Part model, mm, in its own coordinate system. Face numbers are marked on the shaded views. A direction names the side the tool comes from. Round coordinates to 2 decimals unless told otherwise and drop trailing zeros. Order: outer loops, then holes, each group sorted by start corner. A loop starts at its lowest first (then second) coordinate and runs counter-clockwise, first axis right, second up. Notation, with made-up numbers: M 50,1 L 63,1 A22 ccw 63,21 Z; hole C 58.5,-32.5 d7. An arc over 180 degrees is marked long. Write each question's results on one line, items separated by ' | '. Start each with the question number.
1. Band-saw the part on A-A, the plane y = 25. Give the number of separate pieces and of enclosed holes in the cut face, then the cut area to 3 significant figures.
2. Band-saw the part on B-B, the plane x = 107. List the corners of the cut face in (y, z).
3. Band-saw the part on C-C, the plane z = -24. List the corners of the cut face in (x, y).
4. Which spindle directions (+Z, -Z, +X, -X, +Y, -Y) get a long thin tool onto all of the face, cutting with end or side? Do the marked faces 4 and 5. Say none if no direction does.
5. Two-plate mould, pull along Z, no slides. Class the marked faces 1, 2 and 3: +Z half, -Z half, draft (parallel to the pull), parting line (faces both ways), or undercut.
6. Probe L1, parallel to X at y = 13, z = -10.5; L2, parallel to Z at x = 129.5, y = 12; L3, parallel to Z at x = 43, y = 36.5. List the from-to ranges inside material, lowest first. Write a range as [from, to].
7. Drop flat-ended pins along their axis: pin 1 Ø20 at (y, z) = (16, -57.5) entering from -X; pin 2 Ø2.5 at (x, z) = (10.5, -10.5) entering from +Y; pin 3 Ø3 at (x, z) = (-3.5, -42.5) entering from +Y; pin 4 Ø1.8 at (x, z) = (145, -45) entering from -Y. Give the stop position or say it passes through.
```python
from build123d import *

# Parameters (mm, degrees)
SKETCH1_W           = 140
SKETCH1_H           = 90
BOSS_EXTRUDE1_DEPTH = 40
SKETCH2_W           = 135
SKETCH2_H           = 85
CUT_EXTRUDE1_DEPTH  = 37.5
SKETCH3_R           = 3.5
BOSS_EXTRUDE2_DEPTH = 37.5
SKETCH4_R           = 1.5
CUT_EXTRUDE2_DEPTH  = 37.5
BOSS_EXTRUDE3_DEPTH = 3
SKETCH7_R           = 1.5
CUT_EXTRUDE3_DEPTH  = 180.443584449


with BuildPart() as part:
    # Sketch1 → Boss-Extrude1 (new body)
    with BuildSketch(Plane(origin=(0, 0, 0), x_dir=(1, 0, 0), z_dir=(0, 1, 0))):
        with Locations((70, 45)):
            Rectangle(SKETCH1_W, SKETCH1_H)
    extrude(amount=BOSS_EXTRUDE1_DEPTH)

    # Sketch2 → Cut-Extrude1 (cut)
    with BuildSketch(Plane(origin=(0, 40, 0), x_dir=(1, 0, 0), z_dir=(0, 1, 0))):
        with Locations((70, 45)):
            Rectangle(SKETCH2_W, SKETCH2_H)
    extrude(amount=-CUT_EXTRUDE1_DEPTH, mode=Mode.SUBTRACT)

    # Sketch3 → Boss-Extrude2 (add)
    with BuildSketch(Plane(origin=(0, 2.5, 0), x_dir=(1, 0, 0), z_dir=(0, 1, 0))):
        with Locations(Location((10.5, 79.5, 0), (0, 0, 270))):
            Circle(SKETCH3_R)
        with Locations(Location((10.5, 10.5, 0), (0, 0, 270))):
            Circle(SKETCH3_R)
        with Locations(Location((129.5, 10.5, 0), (0, 0, 270))):
            Circle(SKETCH3_R)
        with Locations(Location((129.5, 79.5, 0), (0, 0, 270))):
            Circle(SKETCH3_R)
    extrude(amount=BOSS_EXTRUDE2_DEPTH)

    # Sketch4 → Cut-Extrude2 (cut)
    with BuildSketch(Plane(origin=(0, 40, 0), x_dir=(1, 0, 0), z_dir=(0, 1, 0))):
        with Locations(Location((10.5, 79.5, 0), (0, 0, 270))):
            Circle(SKETCH4_R)
        with Locations(Location((129.5, 79.5, 0), (0, 0, 270))):
            Circle(SKETCH4_R)
        with Locations(Location((10.5, 10.5, 0), (0, 0, 270))):
            Circle(SKETCH4_R)
        with Locations(Location((129.5, 10.5, 0), (0, 0, 270))):
            Circle(SKETCH4_R)
    extrude(amount=-CUT_EXTRUDE2_DEPTH, mode=Mode.SUBTRACT)

    # Sketch5 → Boss-Extrude3 (add)
    with BuildSketch(Plane.XZ):
        with BuildLine():
            ThreePointArc((0, -35), (-7.071067812, -37.928932188), (-10, -45))
            Line((-10, -45), (0, -45))
            Line((0, -45), (0, -35))
        make_face()
        with BuildLine():
            Line((0, -45), (-10, -45))
            ThreePointArc((-10, -45), (-7.071067812, -52.071067812), (0, -55))
            Line((0, -55), (0, -45))
        make_face()
        with BuildLine():
            Line((140, -35), (140, -45))
            Line((140, -45), (150, -45))
            ThreePointArc((150, -45), (147.071067812, -37.928932188), (140, -35))
        make_face()
        with BuildLine():
            Line((150, -45), (140, -45))
            Line((140, -45), (140, -55))
            ThreePointArc((140, -55), (147.071067812, -52.071067812), (150, -45))
        make_face()
    extrude(amount=-BOSS_EXTRUDE3_DEPTH)

    # Sketch7 → Cut-Extrude3 (cut, through all)
    with BuildSketch(Plane.XZ):
        with Locations(Location((-5, -45, 0), (0, 0, 270))):
            Circle(SKETCH7_R)
        with Locations(Location((145, -45, 0), (0, 0, 270))):
            Circle(SKETCH7_R)
    extrude(amount=-CUT_EXTRUDE3_DEPTH, mode=Mode.SUBTRACT)


solid = part.part
```
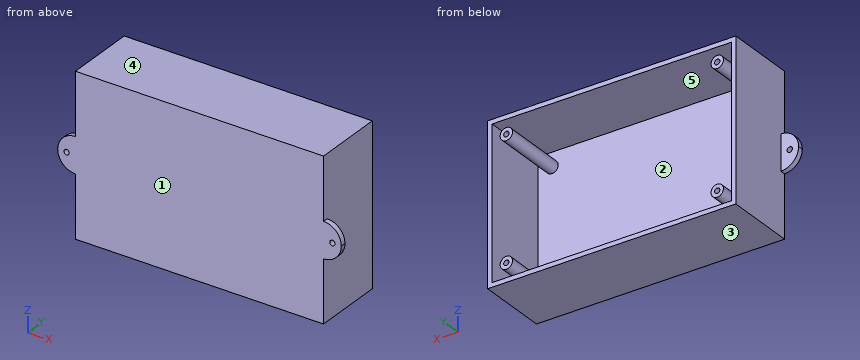
Solution:
1) separate pieces: 5 | enclosed holes: 5 | area: 1,250 mm^2
2) outline: M 0,-90 L 40,-90 L 40,-87.5 L 2.5,-87.5 L 2.5,-2.5 L 40,-2.5 L 40,0 L 0,0 Z
3) outline: M 0,0 L 140,0 L 140,40 L 137.5,40 L 137.5,2.5 L 2.5,2.5 L 2.5,40 L 0,40 Z
4) face 4: +Z, +X, -X, +Y, -Y | face 5: +Y
5) face 1: draft | face 2: undercut | face 3: -Z half
6) L1: [0, 2.5], [7, 9], [12, 14], [126, 128], [131, 133], [137.5, 140] | L2: [-90, -87.5], [-83, -81], [-78, -76], [-14, -12], [-9, -7], [-2.5, 0] | L3: [-90, -87.5], [-2.5, 0]
7) pin 1: x = 0 | pin 2: y = 2.5 | pin 3: y = 3 | pin 4: through
